Geometry check sheet. Reference: the model listing, model coordinates, mm. Face numbers are marked on the shaded views. Round coordinates to 2 decimals unless told otherwise and drop trailing zeros. Loops run counter-clockwise (first coordinate to the right, second up) from the corner with the lowest first, then second, coordinate; pieces in that order, holes last. Notation, with made-up numbers: (20, 87) - (68, 87) arc R12 ccw to (68, 103) - close; hole circle Ø11 at (-8.5, 41). An arc over 180 degrees is marked (long way). Write item = value, one per line.
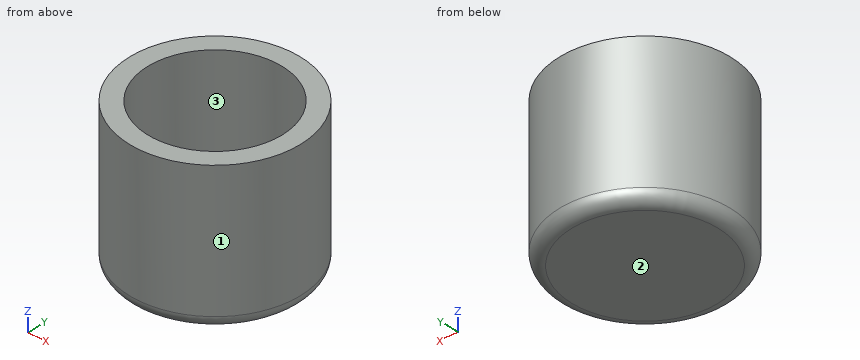
```python
from build123d import *

# Parameters (mm, degrees)
F0_R     = 7
F1_DEPTH = 12
F2_T     = -1.5
F3_R     = 1


with BuildPart() as f1:
    # F0 (on Top) → F1 (new body)
    with BuildSketch(Plane.XY):
        Circle(F0_R)
    extrude(amount=F1_DEPTH)

    # F2
    f2_openings = [f1.faces().sort_by_distance(p)[0] for p in [
        (0, 0, 12),
    ]]
    offset(amount=F2_T, openings=f2_openings)

    # F3
    f3_edges = [f1.edges().sort_by_distance(p)[0] for p in [
        (-7, 0, 0),
    ]]
    fillet(f3_edges, radius=F3_R)


solid = f1.part
```
(1) Gauge pin test, flat ends, axial feed: pin 1 (1.5 mm diameter, centred on x = -4.5, z = 10.5, fed in from -Y); pin 2 (5 mm diameter, centred on y = -1, z = 10.5, fed in from -X); pin 3 (4 mm diameter, centred on y = 4, z = 2.5, fed in from +X); pin 4 (5 mm diameter, centred on x = 4, z = 6.5, fed in from -Y). Record the tip position at first contact, or that the pin passes through.
Answers follow:
pin_1 = -5.91
pin_2 = -7
pin_3 = 6.71
pin_4 = -6.84
(2) Section check A-A (y = 0). Enter the section's corners in (x, z).
Answers follow:
outline = (-7, 1) arc R1 ccw to (-6, 0) - (6, 0) arc R1 ccw to (7, 1) - (7, 12) - (5.5, 12) - (5.5, 1.5) - (-5.5, 1.5) - (-5.5, 12) - (-7, 12) - close
(3) Section check C-C (z = 4.25). Enter the section's corners in (x, y).
Answers follow:
outline = circle Ø14 at (0, 0); hole circle Ø11 at (0, 0)
(4) Mould release check, pull along Y, two halves, no side actions. Record for the marked faces 1, 2 and 3: pulls with the +Y half, pulls with the -Y half, needs draft (parallel to the pull), parting line crosses it, or undercut.
Answers follow:
face_1 = parting line crosses it
face_2 = needs draft
face_3 = undercut
(5) Scan lines: L1, parallel to Y at x = 0, z = 6; L2, parallel to Z at x = -0.25, y = -3.75; L3, parallel to Y at x = -1, z = 5.25. Record each from-to range of solid material in increasing order. Write a range as [from, to].
Answers follow:
L1 = [-7, -5.5], [5.5, 7]
L2 = [0, 1.5]
L3 = [-6.93, -5.41], [5.41, 6.93]
